Read the model definition and answer for the solid it produces. Units are mm, in the model's axes. A direction names the side the tool comes from. Round coordinates to 2 decimals unless told otherwise and drop trailing zeros. Write each loop counter-clockwise with the first axis right and the second up, starting at its lowest first coordinate (ties: lowest second). Pieces come first, ordered by that corner, then holes. Notation, with made-up numbers: (-29, 60) - (-9, 60) arc R24 cw to (-9, 71) - close; hole circle Ø4 at (76.25, 83.5). An arc over 180 degrees is marked (long way). Use one line per item in the form item = value. Start each with the question number.
1) The part is cut by section D-D, the plane y = 2.5. Give the vertices of the cut face in (x, z).
2) This flat-tipped pin is pushed along its axis until it touches: pin 1 (17 mm diameter, centred on x = 15, y = 15, fed in from -Z). Where does it stop, or does it pass through?
3) For faces 5 (the face through (0, -5, 1)), 6 (the face through (0.717, -7.303, 0.986)), 7 (the face through (-29.303, -0.717, 0.986)), 8 (the face through (-27.15, 21.99, 0.99)), determine the directions among +Z, -Z, +X, -X, +Y, -Y from which every point of the face is accessible in a straight line to the end or side of a thin tool.
4) The part is cut by section B-B, the plane z = 0.55. Give the vertices of the cut face in (x, y).
5) The part is cut by section C-C, the plane x = 18.5. Give the vertices of the cut face in (y, z), plus the area to 3 significant figures.
6) For a pull along X with two mould halves and no side action, classify faces 1 (the face through (0, 5, 1)), 2 (the face through (-11, 25, 1)), 3 (the face through (-0.717, 24.303, 0.986)), 4 (the face through (29.283, -0.697, 0.986)) as released by +X, released by -X, zero draft, split by the parting line, or undercut.
7) Consider line 1 along Y through (x, z) = (15, 1.15); line 2 along X through (y, z) = (19.5, 0.9); line 3 along Y through (x, z) = (11, 0.4). Determine where each line is inside the solid, lowest interval first. Write a range as from..to.
8) The part is cut by section A-A, the plane y = 9. Give the vertices of the cut face in (x, z), plus the area to 3 significant figures.
from build123d import *

# Parameters (mm, degrees)
SKETCH1_R           = 7.5
BOSS_EXTRUDE1_DEPTH = 2


with BuildPart() as part:
    # Sketch1 → Boss-Extrude1 (new body)
    with BuildSketch(Plane.XY):
        with BuildLine():
            Line((-20, 25), (-1.414213562, 25))
            Line((-1.414213562, 25), (0, 23.585786438))
            Line((0, 23.585786438), (1.414213562, 25))
            Line((1.414213562, 25), (20, 25))
            ThreePointArc((20, 25), (27.071067812, 22.071067812), (30, 15))
            Line((30, 15), (30, 1.414213562))
            Line((30, 1.414213562), (28.585786438, 0))
            Line((28.585786438, 0), (30, -1.414213562))
            Line((30, -1.414213562), (30, -5))
            ThreePointArc((30, -5), (29.121320344, -7.121320344), (27, -8))
            Line((27, -8), (1.414213562, -8))
            Line((1.414213562, -8), (0, -6.585786438))
            Line((0, -6.585786438), (-1.414213562, -8))
            Line((-1.414213562, -8), (-27, -8))
            ThreePointArc((-27, -8), (-29.121320344, -7.121320344), (-30, -5))
            Line((-30, -5), (-30, -1.414213562))
            Line((-30, -1.414213562), (-28.585786438, 0))
            Line((-28.585786438, 0), (-30, 1.414213562))
            Line((-30, 1.414213562), (-30, 15))
            ThreePointArc((-30, 15), (-27.071067812, 22.071067812), (-20, 25))
        make_face()
        with Locations((15, 15)):
            Circle(SKETCH1_R, mode=Mode.SUBTRACT)
        with Locations(Location((-15, 15, 0), (0, 0, 180))):
            Circle(SKETCH1_R, mode=Mode.SUBTRACT)
        with BuildLine():
            Line((-17.5, 5), (17.5, 5))
            ThreePointArc((17.5, 5), (22.5, 0), (17.5, -5))
            Line((17.5, -5), (-17.5, -5))
            ThreePointArc((-17.5, -5), (-22.5, 0), (-17.5, 5))
        make_face(mode=Mode.SUBTRACT)
    extrude(amount=BOSS_EXTRUDE1_DEPTH)


solid = part.part
Geometry results:
q1.outline = (-30, 0) - (-21.83, 0) - (-21.83, 2) - (-30, 2) - close; (21.83, 0) - (30, 0) - (30, 2) - (21.83, 2) - close
q2.pin_1 = 0
q3.face_5 = +Z, -Z
q3.face_6 = +Z, -Z, -Y
q3.face_7 = +Z, -Z, -X
q3.face_8 = +Z, -Z, -X, +Y
q4.outline = (-30, -5) arc R3 ccw to (-27, -8) - (-1.41, -8) - (0, -6.59) - (1.41, -8) - (27, -8) arc R3 ccw to (30, -5) - (30, -1.41) - (28.59, 0) - (30, 1.41) - (30, 15) arc R10 ccw to (20, 25) - (1.41, 25) - (0, 23.59) - (-1.41, 25) - (-20, 25) arc R10 ccw to (-30, 15) - (-30, 1.41) - (-28.59, 0) - (-30, -1.41) - close; hole circle Ø15 at (-15, 15); hole (-17.5, -5) - (17.5, -5) arc R5 ccw to (17.5, 5) - (-17.5, 5) arc R5 ccw to start; hole circle Ø15 at (15, 15)
q5.outline = (-8, 0) - (-4.9, 0) - (-4.9, 2) - (-8, 2) - close; (4.9, 0) - (8.37, 0) - (8.37, 2) - (4.9, 2) - close; (21.63, 0) - (25, 0) - (25, 2) - (21.63, 2) - close
q5.area = 19.9 mm2
q6.face_1 = undercut
q6.face_2 = zero draft
q6.face_3 = undercut
q6.face_4 = released by +X
q7.line_1 = -8..-5, 5..7.5, 22.5..25
q7.line_2 = -28.93..-21, -9..9, 21..28.93
q7.line_3 = -8..-5, 5..8.66, 21.34..25
q8.outline = (-30, 0) - (-19.5, 0) - (-19.5, 2) - (-30, 2) - close; (-10.5, 0) - (10.5, 0) - (10.5, 2) - (-10.5, 2) - close; (19.5, 0) - (30, 0) - (30, 2) - (19.5, 2) - close
q8.area = 84.0 mm2
